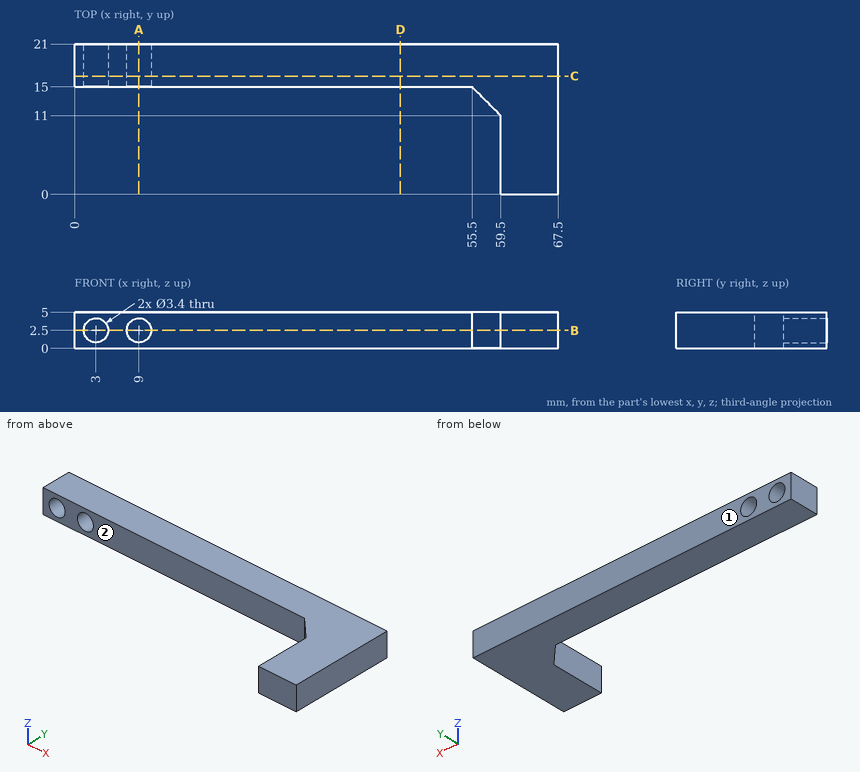
Here's the drawing with two shaded views (mm, measured from the low corner). I have some questions. A direction names the side the tool comes from. Coordinates: 2 decimals unless noted, no trailing zeros. Loops run counter-clockwise (first coordinate to the right, second up) from the corner with the lowest first, then second, coordinate; pieces in that order, holes last.
Item 1: I'm going to push flat-ended pins straight in: pin 1 (3 mm diameter, centred on y = 10, z = 1.5, fed in from -X); pin 2 (2 mm diameter, centred on y = 8, z = 2, fed in from -X); pin 3 (1.5 mm diameter, centred on x = 54.5, z = 3.5, fed in from -Y). Where does each tip first touch, or does it pass through?
Answers below:
pin 1: stops at x = 59
pin 2: stops at x = 59.5
pin 3: stops at y = 15
Item 2: Suppose I cut it at B-B (z = 2.5). Please give me the cut outline in (x, y), then the cut area to 3 significant figures.
Answers below:
outline: (0, 15) - (1.3, 15) - (1.3, 21) - (0, 21) - close; (4.7, 15) - (7.3, 15) - (7.3, 21) - (4.7, 21) - close; (10.7, 15) - (55.5, 15) - (59.5, 11) - (59.5, 0) - (67.5, 0) - (67.5, 21) - (10.7, 21) - close
area: 492 mm2
Item 3: Please list where these lines run through material, in increasing order: L1, parallel to X at y = 17, z = 2.5; L2, parallel to Z at x = 3, y = 16.65; L3, parallel to Y at x = 22, z = 2.3.
Answers below:
L1: x = 0 to 1.3, 4.7 to 7.3, 10.7 to 67.5
L2: z = 0 to 0.8, 4.2 to 5
L3: y = 15 to 21
Item 4: Which directions (+Z, -Z, +X, -X, +Y, -Y) give clear straight access to the entire face, cutting with the end or side of a thin tool? Please do the marked faces 1 and 2.
Answers below:
face 1: +Z, -Z, +X, -X, +Y
face 2: +Z, -Z, -X, -Y
Item 5: Suppose I cut it at A-A (x = 9). Please give me the cut outline in (y, z).
Answers below:
outline: (15, 0) - (21, 0) - (21, 0.8) - (15, 0.8) - close; (15, 4.2) - (21, 4.2) - (21, 5) - (15, 5) - close
Item 6: Suppose I cut it at D-D (x = 45.5). Please give me the cut outline in (y, z), then the cut area to 3 significant figures.
Answers below:
outline: (15, 0) - (21, 0) - (21, 5) - (15, 5) - close
area: 30.0 mm2
Item 7: Suppose I cut it at C-C (y = 16.5). Please give me the cut outline in (x, z).
Answers below:
outline: (0, 0) - (67.5, 0) - (67.5, 5) - (0, 5) - close; hole circle Ø3.4 at (3, 2.5); hole circle Ø3.4 at (9, 2.5)
